```python
from build123d import *

# Parameters (mm, degrees)
BOSS_EXTRUDE1_DEPTH = 3
SKETCH2_W           = 3
SKETCH2_H           = 10
BOSS_EXTRUDE2_DEPTH = 3
SKETCH3_W           = 3
SKETCH3_H           = 3
BOSS_EXTRUDE3_DEPTH = 20
SKETCH4_W           = 3
SKETCH4_H           = 3
BOSS_EXTRUDE4_DEPTH = 10
SKETCH5_W           = 3
SKETCH5_H           = 30
BOSS_EXTRUDE5_DEPTH = 40
SKETCH6_W           = 3
SKETCH6_H           = 30
BOSS_EXTRUDE6_DEPTH = 7


with BuildPart() as part:
    # Sketch1 → Boss-Extrude1 (new body)
    with BuildSketch(Plane.XY):
        with BuildLine():
            ThreePointArc((0, 20), (-5, 15), (0, 10))
            ThreePointArc((0, 10), (10, 0), (0, -10))
            Line((0, -10), (0, -20))
            ThreePointArc((0, -20), (20, 0), (0, 20))
        make_face()
    extrude(amount=BOSS_EXTRUDE1_DEPTH)

    # Sketch2 → Boss-Extrude2 (add)
    with BuildSketch(Plane.ZY):
        with Locations((1.5, -15)):
            Rectangle(SKETCH2_W, SKETCH2_H)
    extrude(amount=-BOSS_EXTRUDE2_DEPTH)

    # Sketch3 → Boss-Extrude3 (add)
    with BuildSketch(Plane(origin=(0, -20, 0), x_dir=(-1, 0, 0), z_dir=(0, -1, 0))):
        with Locations((-1.5, -1.5)):
            Rectangle(SKETCH3_W, SKETCH3_H)
    extrude(amount=-BOSS_EXTRUDE3_DEPTH)

    # Sketch4 → Boss-Extrude4 (add)
    with BuildSketch(Plane.XZ.offset(20)):
        with Locations((1.5, 1.5)):
            Rectangle(SKETCH4_W, SKETCH4_H)
    extrude(amount=BOSS_EXTRUDE4_DEPTH)

    # Sketch5 → Boss-Extrude5 (add)
    with BuildSketch(Plane.XY.offset(3)):
        with Locations((1.5, -15)):
            Rectangle(SKETCH5_W, SKETCH5_H)
    extrude(amount=BOSS_EXTRUDE5_DEPTH)

    # Sketch6 → Boss-Extrude6 (add)
    with BuildSketch(Plane(origin=(0, 0, 0), x_dir=(-1, 0, 0), z_dir=(0, 0, -1))):
        with Locations((-1.5, -15)):
            Rectangle(SKETCH6_W, SKETCH6_H)
    extrude(amount=BOSS_EXTRUDE6_DEPTH)


solid = part.part
```
Design review of the part built by this model. Coordinates are the model's own, in mm. Give positions to 0.01 mm unless a question says otherwise; leave off trailing zeros. Order: outer loops, then holes, each group sorted by start corner. A loop starts at its lowest first (then second) coordinate and runs counter-clockwise, first axis right, second up. Notation, with made-up numbers: M 65.25,82.5 L 120.25,82.5 A28 ccw 120.25,105.5 Z; hole C 51,8 d4. An arc over 180 degrees is marked long. One line per question, with ' | ' between items. Start each with the question number.
Q1. For L1, parallel to X at y = -4.5, z = 39.5; L2, parallel to Y at x = 0.25, z = 17, list the stretches that pass through material, from the lowest coordinate up. Write a range as [from, to].
Q2. We need section A-A (x = 1.75). Write out the cut boundary in (y, z), plus the area to 3 significant figures.
Q3. For pin 1 Ø3.5 at (x, z) = (2, 26) entering from +Y; pin 2 Ø12.5 at (x, y) = (7, 4.5) entering from -Z; pin 3 Ø1.5 at (x, y) = (10.5, 1.5) entering from -Z; pin 4 Ø9 at (y, z) = (-12.5, 12.5) entering from +X, all flat-tipped, find the tip position at first contact; note any pin that passes through.
Q4. We need section D-D (x = 12). Write out the cut boundary in (y, z).
Q5. We need section C-C (z = 24.5). Write out the cut boundary in (x, y).
Q6. We need section B-B (y = -14.5). Write out the cut boundary in (x, z).
Returned:
1) L1: [0, 3] | L2: [-30, 0]
2) outline: M -30,-7 L 0,-7 L 0,43 L -30,43 Z; M 9.85,0 L 19.92,0 L 19.92,3 L 9.85,3 Z | area: 1,530 mm2
3) pin 1: y = 0 | pin 2: z = -7 | pin 3: z = 0 | pin 4: x = 3
4) outline: M -16,0 L 16,0 L 16,3 L -16,3 Z
5) outline: M 0,-30 L 3,-30 L 3,0 L 0,0 Z
6) outline: M 0,-7 L 3,-7 L 3,0 L 13.77,0 L 13.77,3 L 3,3 L 3,43 L 0,43 Z
